from build123d import *

# Parameters (mm, degrees)
F2_DEPTH    = 2
F4_DEPTH    = 2.75
F6_DEPTH    = 2
F7_T2_ANGLE = 111.7162943046
F7_T4_ANGLE = 111.4349059649


# Not quite as in the source:
# - a fillet or chamfer that OpenCascade refuses, or shapes differently, is made with other operations: its cross-section is extruded or revolved along the edge and cut away or added


with BuildPart() as f2:
    # F1 (on Top) → F2 (new body)
    with BuildSketch(Plane.XY):
        with BuildLine():
            ThreePointArc((-12.615433857, -11.3439912447), (-14.7570217863, -7.0788626246), (-15.4994493417, -2.3643613435))
            Line((-15.4994493417, -2.3643613435), (-16.9994473669, -2.3667953738))
            ThreePointArc((-16.9994473669, -2.3667953738), (-16.3370166369, -7.0385981193), (-14.4159247362, -11.34835))
            Line((-14.4159247362, -11.34835), (-12.615433857, -11.3439912447))
        make_face()
        with BuildLine():
            ThreePointArc((-11.9969468723, -11.3424939678), (-14.2251992258, -7.0961265352), (-14.99945, -2.36355))
            Line((-14.99945, -2.36355), (-15.4994493417, -2.3643613435))
            ThreePointArc((-15.4994493417, -2.3643613435), (-14.7570217863, -7.0788626246), (-12.615433857, -11.3439912447))
            Line((-12.615433857, -11.3439912447), (-11.9969468723, -11.3424939678))
        make_face()
        with BuildLine():
            Line((-12.44455, 6.00525), (-14.99945, -2.36355))
            ThreePointArc((-14.99945, -2.36355), (-14.2251992258, -7.0961265352), (-11.9969468723, -11.3424939678))
            Line((-11.9969468723, -11.3424939678), (12.0415, -11.2843))
            ThreePointArc((12.0415, -11.2843), (14.2377010351, -7.0616579823), (15.00045, -2.36355))
            Line((15.00045, -2.36355), (12.58545, 5.79585))
            Line((12.58545, 5.79585), (12.44455, 6.00525))
            Line((12.44455, 6.00525), (5.8368961963, 3.9880080175))
            Line((5.8368961963, 3.9880080175), (5.2849824833, 5.79585))
            Line((5.2849824833, 5.79585), (0, 5.79585))
            Line((0, 5.79585), (-5.2849824833, 5.79585))
            Line((-5.2849824833, 5.79585), (-5.8368961963, 3.9880080175))
            Line((-5.8368961963, 3.9880080175), (-12.44455, 6.00525))
        make_face()
        with BuildLine():
            ThreePointArc((15.00045, -2.36355), (14.2377010351, -7.0616579823), (12.0415, -11.2843))
            Line((12.0415, -11.2843), (12.6599780988, -11.2828027446))
            ThreePointArc((12.6599780988, -11.2828027446), (14.7694777267, -7.043108573), (15.5004493418, -2.3643613211))
            Line((15.5004493418, -2.3643613211), (15.00045, -2.36355))
        make_face()
        with BuildLine():
            ThreePointArc((15.5004493418, -2.3643613211), (14.7694777267, -7.043108573), (12.6599780988, -11.2828027446))
            Line((12.6599780988, -11.2828027446), (14.4604487154, -11.2784440383))
            ThreePointArc((14.4604487154, -11.2784440383), (16.3493648109, -6.9990233555), (17.000447367, -2.3667952845))
            Line((17.000447367, -2.3667952845), (15.5004493418, -2.3643613211))
        make_face()
    extrude(amount=F2_DEPTH)

    # F3 (on face) → F4 (join)
    with BuildSketch(Plane.XY.offset(2)):
        with BuildLine():
            ThreePointArc((-12.615433857, -11.3439912447), (-14.7570217863, -7.0788626246), (-15.4994493417, -2.3643613435))
            Line((-15.4994493417, -2.3643613435), (-16.9994473669, -2.3667953738))
            ThreePointArc((-16.9994473669, -2.3667953738), (-16.3370166369, -7.0385981193), (-14.4159247362, -11.34835))
            Line((-14.4159247362, -11.34835), (-12.615433857, -11.3439912447))
        make_face()
        with BuildLine():
            ThreePointArc((15.5004493418, -2.3643613211), (14.7694777267, -7.043108573), (12.6599780988, -11.2828027446))
            Line((12.6599780988, -11.2828027446), (14.4604487154, -11.2784440383))
            ThreePointArc((14.4604487154, -11.2784440383), (16.3493648109, -6.9990233555), (17.000447367, -2.3667952845))
            Line((17.000447367, -2.3667952845), (15.5004493418, -2.3643613211))
        make_face()
    extrude(amount=F4_DEPTH)

    # F5 (on face) → F6 (join)
    with BuildSketch(Plane.XY.offset(4.75)):
        with BuildLine():
            ThreePointArc((-11.9969468723, -11.3424939678), (-14.2251992258, -7.0961265352), (-14.99945, -2.36355))
            Line((-14.99945, -2.36355), (-15.4994493417, -2.3643613435))
            ThreePointArc((-15.4994493417, -2.3643613435), (-14.7570217863, -7.0788626246), (-12.615433857, -11.3439912447))
            Line((-12.615433857, -11.3439912447), (-11.9969468723, -11.3424939678))
        make_face()
        with BuildLine():
            ThreePointArc((-12.615433857, -11.3439912447), (-14.7570217863, -7.0788626246), (-15.4994493417, -2.3643613435))
            Line((-15.4994493417, -2.3643613435), (-16.9994473669, -2.3667953738))
            ThreePointArc((-16.9994473669, -2.3667953738), (-16.3370166369, -7.0385981193), (-14.4159247362, -11.34835))
            Line((-14.4159247362, -11.34835), (-12.615433857, -11.3439912447))
        make_face()
        with BuildLine():
            Line((-12.9994526331, -2.3603046262), (-14.99945, -2.36355))
            ThreePointArc((-14.99945, -2.36355), (-14.2251992258, -7.0961265352), (-11.9969468723, -11.3424939678))
            Line((-11.9969468723, -11.3424939678), (-9.3831293237, -11.3361662539))
            ThreePointArc((-9.3831293237, -11.3361662539), (-12.0576120471, -7.1972712434), (-12.9994526331, -2.3603046262))
        make_face()
        with BuildLine():
            ThreePointArc((13.000452633, -2.3603047155), (12.0703811691, -7.1680366652), (9.4277378752, -11.2906275797))
            Line((9.4277378752, -11.2906275797), (12.0415, -11.2843))
            ThreePointArc((12.0415, -11.2843), (14.2377010351, -7.0616579823), (15.00045, -2.36355))
            Line((15.00045, -2.36355), (13.000452633, -2.3603047155))
        make_face()
        with BuildLine():
            ThreePointArc((15.00045, -2.36355), (14.2377010351, -7.0616579823), (12.0415, -11.2843))
            Line((12.0415, -11.2843), (14.4604487154, -11.2784440383))
            ThreePointArc((14.4604487154, -11.2784440383), (16.3493648109, -6.9990233555), (17.000447367, -2.3667952845))
            Line((17.000447367, -2.3667952845), (15.00045, -2.36355))
        make_face()
    extrude(amount=F6_DEPTH)

    # F7: chamfer of 3 on 2 edges, made by hand

    # F7_s1 → F7_t2 (revolve, cut)
    with BuildSketch(Plane(origin=(0.4833612439, -0.1044854652, 0), x_dir=(0, 0, 1), z_dir=(0.9774246375, -0.2112843535, 0))):
        Polygon((3.75, 15.2861027758), (6.75, 18.2861027758), (6.75, 15.2861027758), align=None)
    revolve(axis=Axis((0.0002934681, -2.3392100804, 6.75), (0, 0, -1)), revolution_arc=F7_T2_ANGLE, mode=Mode.SUBTRACT)

    # F7_s3 → F7_t4 (revolve, cut)
    with BuildSketch(Plane(origin=(1.0831916717, -1.6111813469, 0), x_dir=(0, 0, 1), z_dir=(-0.5579305881, 0.8298876182, 0))):
        Polygon((6.75, 14.695302969), (3.75, 11.695302969), (6.75, 11.695302969), align=None)
    revolve(axis=Axis((0.0002934681, -2.3392100804, 6.75), (0, 0, -1)), revolution_arc=F7_T4_ANGLE, mode=Mode.SUBTRACT)


solid = f2.part
Geometry: final body of the model. Coordinates: model frame, mm. A direction names the side the tool comes from. Round coordinates to 2 decimals unless told otherwise and drop trailing zeros. Loops run counter-clockwise (first coordinate to the right, second up) from the corner with the lowest first, then second, coordinate; pieces in that order, holes last.
Q1. Section B-B on y = 4.75. Return loops of the section in (x, z) (3 decimals).
Q2. Pin query (flat end, axial travel): P1, Ø1, axis at y = -6, z = 1.5, coming from the +X side; P2, Ø1.6, axis at x = -2, z = 1.5, coming from the +Y side; P3, Ø3, axis at x = -12.5, z = 6, coming from the -Y side; P4, Ø8, axis at x = 13, y = 1, coming from the +Z side. Return the tip coordinate at first contact, or that it passes through.
Q3. Section A-A on z = 3.75. Return loops of the section in (x, y).
Q4. Section C-C on z = 1.5. Return loops of the section in (x, y), plus the area to 3 significant figures.
Q5. Access query for faces 1 (the conical face through (13.906, -7.3, 5.514)), 2 (the cylindrical face through (14.79, -6.98, 3.36)), 3 (the flat face through (5.565, 4.879, 0.986)), 4 (the flat face through (-16, -7, 6.75)). Directions: +Z, -Z, +X, -X, +Y, -Y. A direction counts if a zero-diameter tool reaches every point of the face in a straight line with its end or side. Return the directions, or none.
Q6. Section D-D on x = -4. Return loops of the section in (y, z), plus the area to 3 significant figures.
Q7. Pull-direction query (Z, two-part tool) for faces 5 (the flat face through (0, -3, 0)), 6 (the flat face through (-14, -7, 4.75)), 7 (the cylindrical face through (-16.355, -6.975, 3.328)), 8 (the conical face through (-13.87, -7.48, 5.54)); classes: released by +Z, released by -Z, zero draft, split by the parting line, or undercut.
Q8. Material intervals for L1, parallel to Z at x = 0.5, y = 4.25; L2, parallel to X at y = -5.5, z = 3.5; L3, parallel to X at y = -6.5, z = 5, sorted ascending.
Evaluation:
1. outline: (-12.828, 0) - (-8.333, 0) - (-8.333, 2) - (-12.828, 2) - close; (-5.604, 0) - (5.604, 0) - (5.604, 2) - (-5.604, 2) - close; (8.333, 0) - (12.895, 0) - (12.895, 2) - (8.333, 2) - close
2. P1: stops at x = 16.7
2. P2: stops at y = 5.8
2. P3: stops at y = -11.35
2. P4: stops at z = 5.91
3. outline: (-17, -2.37) arc R17 ccw to (-14.42, -11.35) - (-12.62, -11.34) arc R15.5 cw to (-15.5, -2.36) - close; (12.66, -11.28) - (14.46, -11.28) arc R17 ccw to (17, -2.37) - (15.5, -2.36) arc R15.5 cw to start
4. outline: (-17, -2.37) arc R17 ccw to (-14.42, -11.35) - (14.46, -11.28) arc R17 ccw to (17, -2.37) - (15, -2.36) - (12.59, 5.8) - (12.44, 6.01) - (5.84, 3.99) - (5.28, 5.8) - (-5.28, 5.8) - (-5.84, 3.99) - (-12.44, 6.01) - (-15, -2.36) - close
4. area: 503 mm2
5. face 1: +Z, +Y
5. face 2: +Y
5. face 3: +Z, -Z, +Y
5. face 4: +Z, +X, -X, +Y, -Y
6. outline: (-11.32, 0) - (5.8, 0) - (5.8, 2) - (-11.32, 2) - close
6. area: 34.2 mm2
7. face 5: released by -Z
7. face 6: undercut
7. face 7: zero draft
7. face 8: released by +Z
8. L1: z = 0 to 2
8. L2: x = -16.7 to -15.17, 15.17 to 16.7
8. L3: x = -16.48 to -13.63, 13.63 to 16.48
